Source: CAD feature listing. Evaluate the final solid. Frame: model axes, mm. A direction names the side the tool comes from. Give positions to 0.01 mm unless a question says otherwise; leave off trailing zeros. Order: outer loops, then holes, each group sorted by start corner. A loop starts at its lowest first (then second) coordinate and runs counter-clockwise, first axis right, second up.
from build123d import *

# Parameters (mm, degrees)
SKETCH_W        = 17
SKETCH_H        = 31
PAD_DEPTH       = 38
SKETCH002_W     = 13
SKETCH002_H     = 13
POCKET001_DEPTH = 36
SKETCH003_W     = 4.2
SKETCH003_H     = 4.2
POCKET002_DEPTH = 5
SKETCH001_W     = 13
SKETCH001_H     = 2
POCKET_DEPTH    = 36
SKETCH004_W     = 6
SKETCH004_H     = 30
POCKET003_DEPTH = 7.5
SKETCH006_W     = 6
SKETCH006_H     = 30
POCKET004_DEPTH = 7.5
SKETCH007_R     = 2
POCKET005_DEPTH = 5
SKETCH008_R     = 2
POCKET006_DEPTH = 2


with BuildPart() as part:
    # Sketch → Pad (new body)
    with BuildSketch(Plane.XY):
        with Locations((8.5, 15.5)):
            Rectangle(SKETCH_W, SKETCH_H)
    extrude(amount=PAD_DEPTH)

    # Sketch002 (on DatumPlane) → Pocket001 (cut)
    with BuildSketch(Plane.XY.offset(38)):
        with Locations((8.5, 8.5)):
            Rectangle(SKETCH002_W, SKETCH002_H)
    extrude(amount=-POCKET001_DEPTH, mode=Mode.SUBTRACT)

    # Sketch003 (on DatumPlane) → Pocket002 (cut)
    with BuildSketch(Plane(origin=(0, 0, 0), x_dir=(1, 0, 0), z_dir=(0, 0, -1))):
        with Locations((8.5, -8.5)):
            Rectangle(SKETCH003_W, SKETCH003_H)
    extrude(amount=-POCKET002_DEPTH, mode=Mode.SUBTRACT)

    # Sketch001 (on DatumPlane) → Pocket (cut)
    with BuildSketch(Plane.XY.offset(38)):
        with Locations((8.5, 20)):
            Rectangle(SKETCH001_W, SKETCH001_H)
    extrude(amount=-POCKET_DEPTH, mode=Mode.SUBTRACT)

    # Sketch004 (on DatumPlane) → Pocket003 (cut)
    with BuildSketch(Plane(origin=(0, 0, 0), x_dir=(0, -1, 0), z_dir=(-1, 0, 0))):
        with Locations((-26, 17)):
            Rectangle(SKETCH004_W, SKETCH004_H)
    extrude(amount=-POCKET003_DEPTH, mode=Mode.SUBTRACT)

    # Sketch006 (on DatumPlane) → Pocket004 (cut)
    with BuildSketch(Plane.YZ.offset(17)):
        with Locations((26, 17)):
            Rectangle(SKETCH006_W, SKETCH006_H)
    extrude(amount=-POCKET004_DEPTH, mode=Mode.SUBTRACT)

    # Sketch007 (on DatumPlane) → Pocket005 (cut)
    with BuildSketch(Plane.XZ.offset(-15)):
        with Locations((5.5, 31)):
            Circle(SKETCH007_R)
        with Locations((11.5, 31)):
            Circle(SKETCH007_R)
        with Locations((5.5, 5)):
            Circle(SKETCH007_R)
        with Locations((11.5, 5)):
            Circle(SKETCH007_R)
    extrude(amount=-POCKET005_DEPTH, mode=Mode.SUBTRACT)

    # Sketch008 (on DatumPlane) → Pocket006 (cut)
    with BuildSketch(Plane(origin=(0, 23, 0), x_dir=(-1, 0, 0), z_dir=(0, 1, 0))):
        with Locations((-5.5, 18)):
            Circle(SKETCH008_R)
        with Locations((-11.5, 18)):
            Circle(SKETCH008_R)
    extrude(amount=-POCKET006_DEPTH, mode=Mode.SUBTRACT)


solid = part.part
1) Section query D-D on z = 9.5. Output: boundary loops of the cut face in (x, y).
Checks:
outline: (0, 0) - (17, 0) - (17, 23) - (9.5, 23) - (9.5, 29) - (17, 29) - (17, 31) - (0, 31) - (0, 29) - (7.5, 29) - (7.5, 23) - (0, 23) - close; hole (2, 2) - (15, 2) - (15, 15) - (2, 15) - close; hole (2, 19) - (15, 19) - (15, 21) - (2, 21) - close
2) Section query A-A on z = 5. Output: boundary loops of the cut face in (x, y).
Checks:
outline: (0, 0) - (17, 0) - (17, 23) - (9.5, 23) - (9.5, 29) - (17, 29) - (17, 31) - (0, 31) - (0, 29) - (7.5, 29) - (7.5, 23) - (0, 23) - close; (7.5, 15) - (9.5, 15) - (9.5, 19) - (7.5, 19) - close; hole (2, 2) - (15, 2) - (15, 15) - (13.5, 15) - (13.5, 19) - (15, 19) - (15, 21) - (2, 21) - (2, 19) - (3.5, 19) - (3.5, 15) - (2, 15) - close
3) Reachability of faces 1 (the face through (7.5, 26, 17)), 2 (the face through (3.502, 16.972, 5.088)), 3 (the face through (6.4, 9, 1)), 4 (the face through (13.3, 23, 16.8)), 5 (the face through (15, 20, 20)) from +Z, -Z, +X, -X, +Y, -Y: full face, straight path, thin tool, end or side. Return the list, or none.
Checks:
face 1: -X
face 2: none
face 3: +Z, -Z
face 4: +X
face 5: +Z
4) Section query B-B on x = 2.5. Output: boundary loops of the cut face in (y, z).
Checks:
outline: (0, 0) - (31, 0) - (31, 38) - (21, 38) - (21, 2) - (19, 2) - (19, 38) - (15, 38) - (15, 2) - (2, 2) - (2, 38) - (0, 38) - close; hole (23, 2) - (29, 2) - (29, 32) - (23, 32) - close
5) Ray query, L1, parallel to Y at x = 14.75, z = 13; L2, parallel to Z at x = 11.5, y = 16.65; L3, parallel to Y at x = 5, z = 4.5. Return the intervals inside material, ascending.
Checks:
L1: y = 0 to 2, 15 to 19, 21 to 23, 29 to 31
L2: z = 0 to 3, 7 to 29, 33 to 38
L3: y = 0 to 2, 21 to 23, 29 to 31
6) Section query C-C on y = 9. Output: boundary loops of the cut face in (x, z), and give its area (3 significant figures).
Checks:
outline: (0, 0) - (6.4, 0) - (6.4, 2) - (2, 2) - (2, 38) - (0, 38) - close; (10.6, 0) - (17, 0) - (17, 38) - (15, 38) - (15, 2) - (10.6, 2) - close
area: 170 mm2
7) Pull-direction query (X, two-part tool) for faces 6 (the face through (17, 15, 19)), 7 (the face through (9.502, 16.972, 5.088)), 8 (the face through (4, 26, 32)); classes: +X half, -X half, draft (parallel to the pull), parting line (faces both ways), or undercut.
Checks:
face 6: +X half
face 7: undercut
face 8: draft
8) First-contact query: pin 1 Ø0.6 at (x, y) = (9, 19.5) entering from +Z; pin 2 Ø1.8 at (y, z) = (26.5, 20.5) entering from -X. Flat tips, straight axial feed; report the tip coordinate or a pass-through.
Checks:
pin 1: stops at z = 2
pin 2: stops at x = 7.5
